Build history of the part. All positions in model axes, mm. A direction names the side the tool comes from. Give positions to 0.01 mm unless a question says otherwise; leave off trailing zeros. Write each loop counter-clockwise with the first axis right and the second up, starting at its lowest first coordinate (ties: lowest second). Pieces come first, ordered by that corner, then holes. Notation, with made-up numbers: (66.25, 76.25) -> (109.25, 76.25) arc R29 ccw to (109.25, 113.25) -> close; hole circle Ø2 at (28.5, 79.5). An arc over 180 degrees is marked (long way). Write item = value, one per line. Start each with the question number.
Q1. Saw through at D-D, the plane x = 10.5. List the corners of the cut face in (y, z), then the cut area to 3 significant figures.
Q2. Mould opens along Z. For faces 1 (the face through (-19.05, 43.64, -10.39)), 2 (the face through (-19.05, 56.21, 10.64)), 3 (the face through (19.05, 44.06, 36.28)), 4 (the face through (12.66, 1.18, -24.82)) say: pulls with the +Z half, pulls with the -Z half, needs draft (parallel to the pull), parting line crosses it, or undercut.
Q3. Tool access for faces 5 (the face through (-19.051, 48.09, 43.753)), 6 (the face through (-0.29, 27.46, 49.41)), 7 (the face through (19.051, 34.753, -7.433)), 8 (the face through (19.051, 0.344, 31.575)), 9 (the face through (19.05, 43.64, -10.39)): list every direction of +Z, -Z, +X, -X, +Y, -Y with a clear straight run to the whole face (end or side of a thin tool).
Q4. Drop flat-ended pins along their axis: P1, Ø10.5, axis at x = -1.5, z = -8, coming from the +Y side; P2, Ø10.5, axis at y = 14.87, z = 19.32, coming from the -X side; P3, Ø8, axis at x = -13.5, y = 42.5, coming from the -Z side; P4, Ø0.7, axis at x = 2, y = 1.5, coming from the +Z side. Give the stop position or say it passes through.
Q5. Wall check: line 1 (X direction, y = 44, z = 53); line 2 (Y direction, x = 14, z = -18); line 3 (Z direction, x = 15, y = 43). Give the ranges that are in metal, low to high.
Q6. Saw through at A-A, the plane x = 2. List the corners of the cut face in (y, z), then the cut area to 3 significant figures.
Q7. Saw through at B-B, the plane y = 13.5. List the corners of the cut face in (x, z), then the cut area to 3 significant figures.
Q8. Saw through at C-C, the plane z = 20. List the corners of the cut face in (x, y), then the cut area to 3 significant figures.
from build123d import *

# Parameters (mm, degrees)
SKETCH1_W           = 35.56
SKETCH1_H           = 63.5
SKETCH1_R           = 3.0734
BOSS_EXTRUDE1_DEPTH = 2.4003
SKETCH2_R           = 4.07035
BOSS_EXTRUDE2_DEPTH = 2.5781
SKETCH3_W           = 40.7162
SKETCH3_H           = 18.5166
BOSS_EXTRUDE3_DEPTH = 2.54
SKETCH4_R           = 5.5626
BOSS_EXTRUDE4_DEPTH = 3.7846


with BuildPart() as part:
    # Sketch1 → Boss-Extrude1 (new body)
    with BuildSketch(Plane(origin=(0, 0, 0), x_dir=(1, 0, 0), z_dir=(0, 1, 0))):
        Rectangle(SKETCH1_W, SKETCH1_H)
        with Locations((-11.0109, 22.225)):
            Circle(SKETCH1_R, mode=Mode.SUBTRACT)
        with Locations((-11.0109, -18.288)):
            Circle(SKETCH1_R, mode=Mode.SUBTRACT)
        with Locations((11.0109, -18.288)):
            Circle(SKETCH1_R, mode=Mode.SUBTRACT)
        with Locations((11.0109, 22.225)):
            Circle(SKETCH1_R, mode=Mode.SUBTRACT)
    extrude(amount=BOSS_EXTRUDE1_DEPTH)

    # Sketch2 → Boss-Extrude2 (add)
    with BuildSketch(Plane(origin=(17.78, 0, 0), x_dir=(0, 0, -1), z_dir=(1, 0, 0))):
        with BuildLine():
            Line((31.75, 0), (31.75, 5.119118053))
            ThreePointArc((31.75, 5.119118053), (31.680088236, 5.710949198), (31.474201493, 6.270200848))
            Line((31.474201493, 6.270200848), (17.693567666, 33.376966591))
            ThreePointArc((17.693567666, 33.376966591), (16.006303844, 34.699493087), (13.908046107, 34.259890987))
            Line((13.908046107, 34.259890987), (13.489778208, 33.947050723))
            ThreePointArc((13.489778208, 33.947050723), (7.374615324, 34.828872577), (8.256437178, 40.944035461))
            Line((8.256437178, 40.944035461), (9.378285973, 41.783113656))
            ThreePointArc((9.378285973, 41.783113656), (10.39301658, 43.675533493), (9.59524257, 45.66914521))
            ThreePointArc((9.59524257, 45.66914521), (-10.963994808, 56.277959645), (-34.028081087, 54.467680828))
            ThreePointArc((-34.028081087, 54.467680828), (-35.535691357, 52.940715566), (-35.336051172, 50.80421014))
            Line((-35.336051172, 50.80421014), (-34.816573654, 49.916114029))
            ThreePointArc((-34.816573654, 49.916114029), (-36.36360729, 44.008751256), (-42.270970063, 45.555784893))
            Line((-42.270970063, 45.555784893), (-45.277675805, 50.696033664))
            ThreePointArc((-45.277675805, 50.696033664), (-46.831353511, 51.871946179), (-48.760952094, 51.601143727))
            Line((-48.760952094, 51.601143727), (-56.540301411, 47.010806757))
            ThreePointArc((-56.540301411, 47.010806757), (-57.70907124, 45.457347112), (-57.437054463, 43.532440191))
            Line((-57.437054463, 43.532440191), (-32.487107654, 1.249193243))
            ThreePointArc((-32.487107654, 1.249193243), (-31.559101504, 0.334297259), (-30.299547846, 0))
            Line((-30.299547846, 0), (31.75, 0))
        make_face()
        with Locations((-19.316644044, 14.86535)):
            Circle(SKETCH2_R, mode=Mode.SUBTRACT)
    boss_extrude2 = extrude(amount=BOSS_EXTRUDE2_DEPTH)

    # Mirror1: Boss-Extrude2 across plane
    add(boss_extrude2.mirror(Plane.ZY))

    # Sketch3 → Boss-Extrude3 (add)
    with BuildSketch(Plane(origin=(0, -13.896244991, 23.550285021), x_dir=(1, 0, 0), z_dir=(0, -0.508191637, 0.861244019))):
        with Locations((0, 58.016828481)):
            Rectangle(SKETCH3_W, SKETCH3_H)
    extrude(amount=BOSS_EXTRUDE3_DEPTH)

    # Sketch4 → Boss-Extrude4 (add)
    with BuildSketch(Plane(origin=(0, -13.896244991, 23.550285021), x_dir=(-1, 0, 0), z_dir=(0, 0.508191637, -0.861244019))):
        with Locations((0, 58.016828481)):
            Circle(SKETCH4_R)
    extrude(amount=BOSS_EXTRUDE4_DEPTH)


solid = part.part
Report:
q1.outline = (0, -31.75) -> (2.4, -31.75) -> (2.4, -25.26) -> (0, -25.26) -> close; (0, -19.19) -> (2.4, -19.19) -> (2.4, 15.26) -> (0, 15.26) -> close; (0, 21.32) -> (2.4, 21.32) -> (2.4, 31.75) -> (0, 31.75) -> close; (26.81, 50.52) -> (28.1, 48.33) -> (44.04, 57.74) -> (42.75, 59.93) -> close
q1.area = 170 mm2
q2.face_1 = pulls with the -Z half
q2.face_2 = parting line crosses it
q2.face_3 = undercut
q2.face_4 = undercut
q3.face_5 = +X, -X, +Y
q3.face_6 = +X, -X, -Y
q3.face_7 = +X, -X
q3.face_8 = +Z, +X, -Y
q3.face_9 = -Z, +X, -X
q4.P1 = 2.4
q4.P2 = -20.36
q4.P3 = 54.47
q4.P4 = 31.75
q5.line_1 = -20.36 to -17.78, 17.78 to 20.36
q5.line_2 = 0 to 2.4
q5.line_3 = 57.12 to 59.51
q6.outline = (0, -31.75) -> (2.4, -31.75) -> (2.4, 31.75) -> (0, 31.75) -> close; (26.81, 50.52) -> (28.1, 48.33) -> (31.6, 50.4) -> (33.52, 47.14) -> (42.46, 52.41) -> (40.54, 55.67) -> (44.04, 57.74) -> (42.75, 59.93) -> close
q6.area = 239 mm2
q7.outline = (-20.36, -27.8) -> (-17.78, -27.8) -> (-17.78, 15.48) -> (-20.36, 15.48) -> close; (-20.36, 23.15) -> (-17.78, 23.15) -> (-17.78, 39.72) -> (-20.36, 39.72) -> close; (17.78, -27.8) -> (20.36, -27.8) -> (20.36, 15.48) -> (17.78, 15.48) -> close; (17.78, 23.15) -> (20.36, 23.15) -> (20.36, 39.72) -> (17.78, 39.72) -> close
q7.area = 309 mm2
q8.outline = (-20.36, 0) -> (-13.56, 0) -> (-13.56, 2.4) -> (-17.78, 2.4) -> (-17.78, 10.85) -> (-20.36, 10.85) -> close; (-20.36, 18.88) -> (-17.78, 18.88) -> (-17.78, 57.11) -> (-20.36, 57.11) -> close; (-8.46, 0) -> (8.46, 0) -> (8.46, 2.4) -> (-8.46, 2.4) -> close; (13.56, 0) -> (20.36, 0) -> (20.36, 10.85) -> (17.78, 10.85) -> (17.78, 2.4) -> (13.56, 2.4) -> close; (17.78, 18.88) -> (20.36, 18.88) -> (20.36, 57.11) -> (17.78, 57.11) -> close
q8.area = 314 mm2
